Solid Edge part; units mm, degrees
sketch "Sketch1" plane through (0, 0, 0) normal (0, 0, 1) x (1, 0, 0)
  line L0 (0, 50) -> (0, -50)
  arc A0 (0, 50) -> (0, -50) centre (0, 0) cw
extrude "Protrusion1" add sketch "Sketch1" along normal blind 25
sketch "Sketch2" plane through (0, 0, 0) normal (0, -1, 0) x (1, 0, 0)
  line L0 (-45, 70) -> (-15, 70)
  arc A0 (25, 30) -> (-15, 70) centre (25, 70) cw
  line L1 (25, 0) -> (25, 30)
  arc A1 (25, 0) -> (-45, 70) centre (25, 70) cw
extrude "ExtrudedProtrusion_2" add sketch "Sketch2" along normal mid plane 30
sketch "Sketch3" plane through (0, 0, 0) normal (1, 0, 0) x (0, 1, 0)
  line L0 (-5, 70) -> (-5, 46)
  line L1 (-5, 46) -> (5, 46)
  line L2 (5, 46) -> (5, 70)
extrude "Cutout1" cut sketch "Sketch3" against normal up to next material side at (0, -4.95, 58)
sketch "Sketch4" plane through (0, 0, 0) normal (0, -1, 0) x (1, 0, 0)
  line L0 (50, 25) -> (32, 25)
  line L1 (32, 25) -> (32, 20)
  line L2 (32, 20) -> (50, 20)
  line L3 (50, 20) -> (50, 25)
extrude "Cutout2" cut sketch "Sketch4" along normal mid plane 30
Build history of the part. All positions in model axes, mm. A direction names the side the tool comes from. Coordinates: 2 decimals unless noted, no trailing zeros. Order: outer loops, then holes, each group sorted by start corner. A loop starts at its lowest first (then second) coordinate and runs counter-clockwise, first axis right, second up.
Item 1: Drill centre lines: L1, parallel to Y at x = -21, z = 52; L2, parallel to Y at x = -2.5, z = 7; L3, parallel to Z at x = 7.5, y = 39. Where is each one in solid material? Low to high.
Filled in:
L1: y = -15 to -5, 5 to 15
L2: y = -15 to 15
L3: z = 0 to 25
Item 2: Saw through at D-D on z = 28. List the corners of the cut face in (x, y).
Filled in:
outline: (-31, -15) - (25, -15) - (25, 15) - (-31, 15) - close
Item 3: Drop flat-ended pins along their axis: pin 1 Ø2.5 at (x, z) = (36.5, 23) entering from +Y; pin 2 Ø5.5 at (y, z) = (-2.5, 28) entering from +X; pin 3 Ø3 at (x, y) = (-26.5, 0) entering from +Z. Give the stop position or say it passes through.
Filled in:
pin 1: stops at y = 35.46
pin 2: stops at x = 25
pin 3: stops at z = 46
Item 4: Saw through at B-B on x = 34.5. List the corners of the cut face in (y, z), then the cut area to 3 significant figures.
Filled in:
outline: (-36.19, 0) - (36.19, 0) - (36.19, 25) - (15, 25) - (15, 20) - (-15, 20) - (-15, 25) - (-36.19, 25) - close
area: 1,660 mm2
Item 5: Saw through at A-A on y = 0. List the corners of the cut face in (x, z), then the cut area to 3 significant figures.
Filled in:
outline: (-40.76, 46) arc R70 ccw to (0, 4.62) - (0, 0) - (50, 0) - (50, 20) - (32, 20) - (32, 25) - (25, 25) - (25, 30) arc R40 cw to (-7, 46) - close
area: 2,420 mm2
Item 6: Tool access for faces 1 (the flat face through (25, 0, 27)), 2 (the flat face through (32, 0, 23)), 3 (the flat face through (-24, 0, 46)): list every direction of +Z, -Z, +X, -X, +Y, -Y with a clear straight run to the whole face (end or side of a thin tool).
Filled in:
face 1: +Z, +X, +Y, -Y
face 2: +Z, +X
face 3: +Z, +X, -X
Item 7: Saw through at C-C on z = 55. List the corners of the cut face in (x, y), then the cut area to 3 significant figures.
Filled in:
outline: (-43.37, -15) - (-12.08, -15) - (-12.08, -5) - (-43.37, -5) - close; (-43.37, 5) - (-12.08, 5) - (-12.08, 15) - (-43.37, 15) - close
area: 626 mm2
